The model under review builds one solid part; all positions refer to its coordinate system, in mm. A direction names the side the tool comes from. Round coordinates to 2 decimals unless told otherwise and drop trailing zeros. Order: outer loops, then holes, each group sorted by start corner. A loop starts at its lowest first (then second) coordinate and runs counter-clockwise, first axis right, second up. Notation, with made-up numbers: M 76,48 L 86,48 A20 ccw 86,52 Z; hole C -5.75,-30 d9. An arc over 180 degrees is marked long. One line per item, written item: value. Start each with the question number.
from build123d import *

# Parameters (mm, degrees)
BOSS_EXTRUDE1_DEPTH = 50.8
SKETCH14_W          = 60.289388783
SKETCH14_H          = 44.45


with BuildPart() as part:
    # Sketch1 → Boss-Extrude1 (new body)
    with BuildSketch(Plane.XY):
        Polygon((-6.329511048, -89.779515299), (-184.2678796, 104.406138968), (-115.365720991, 104.406138968), (16.023023921, -38.979515299), (-6.329511048, -38.979515299), align=None)
    extrude(amount=BOSS_EXTRUDE1_DEPTH)

    # Cut-Sweep1: sweep along a path in Sketch13
    with BuildLine(Plane.XY.offset(25.4)) as cut_sweep1_path:
        Line((-149.816800296, 104.406138968), (41.274977184, -104.133942279))
    # Sketch14 → Cut-Sweep1 (sweep, cut)
    with BuildSketch(Plane(origin=(0, 104.406138968, 0), x_dir=(1, 0, 0), z_dir=(0, 1, 0))):
        with Locations((-149.816800296, -25.4)):
            Rectangle(SKETCH14_W, SKETCH14_H)
    sweep(path=cut_sweep1_path.line, mode=Mode.SUBTRACT)


solid = part.part
Item 1: Consider section C-C, the plane y = 55. Give the boundary of the cut face in (x, z) (1 decimal).
Item 2: Machinability: for faces 1 (the flat face through (-6.33, -87, 29)), 2 (the flat face through (-76, 29, 50.8)), 3 (the flat face through (-77, 30, 3.175)), which of the approach directions +Z, -Z, +X, -X, +Y, -Y give a long, thin tool a straight path to every point of the face, cutting with its end or side? Answer none if there is none.
Item 3: Wall thickness on L1, parallel to Z at x = -88, y = 8.5 (3 decimals); L2, parallel to Y at x = -116.5, z = 38; L3, parallel to Y at x = -63, z = 44: over which ranges is each line inside the solid? List them lowest first.
Item 4: Consider section A-A, the plane z = 26.5. Give the boundary of the cut face in (x, y).
Item 5: Clearance check with flat-ended pins moving along their axes: P1, Ø6, axis at y = 47.5, z = 6.5, coming from the +X side; P2, Ø8, axis at x = -57, z = 38.5, coming from the -Y side; P3, Ø5, axis at x = -44, z = 7.5, coming from the -Y side. State where each tip first meets the part, or that it passes through.
Item 6: Consider section B-B, the plane x = -85. Give the boundary of the cut face in (y, z) (3 decimals), then the cut area to 3 significant figures.
Item 7: The part is to be moulded in two halves that separate along Z. For faces 4 (the flat face through (-76, 29, 0)), 5 (the flat face through (-150, 104.406, 3)), 6 (the flat face through (-77, 30, 47.625)), 7 (the flat face through (-91.93, 8.337, 25.089)), say which applies: pulls with the +Z half, pulls with the -Z half, needs draft (parallel to the pull), parting line crosses it, or undercut.
Item 8: Consider section D-D, the plane y = -42.5. Give the boundary of the cut face in (x, z) (3 decimals).
Computed:
1. outline: M -139,0 L -70.1,0 L -70.1,50.8 L -139,50.8 Z; hole M -134.7,3.2 L -74.4,3.2 L -74.4,47.6 L -134.7,47.6 Z
2. face 1: +Z, -Z, +X, -Y
2. face 2: +Z, +X, -X, +Y, -Y
2. face 3: none
3. L1: z = 0 to 3.175, 47.625 to 50.8
3. L2: y = 30.45 to 35.15, 100.94 to 104.41
3. L3: y = -27.93 to -23.23, 42.56 to 47.26
4. outline: M -184.27,104.41 L -6.33,-89.78 L -6.33,-85.08 L -179.96,104.41 Z; M -119.67,104.41 L 11.72,-38.98 L 16.02,-38.98 L -115.37,104.41 Z
5. P1: stops at x = -60.47
5. P2: stops at y = -38.85
5. P3: stops at y = -51.4
6. outline: M -3.926,0 L 71.268,0 L 71.268,50.8 L -3.926,50.8 Z; hole M 0.774,3.175 L 66.568,3.175 L 66.568,47.625 L 0.774,47.625 Z
6. area: 895 mm^2
7. face 4: pulls with the -Z half
7. face 5: needs draft
7. face 6: undercut
7. face 7: undercut
8. outline: M -49.653,0 L -6.33,0 L -6.33,3.175 L -45.347,3.175 L -45.347,47.625 L -6.33,47.625 L -6.33,50.8 L -49.653,50.8 Z
